```python
from build123d import *

# Parameters (mm, degrees)
BOSS_EXTRUDE1_DEPTH = 2
FILLET1_R           = 1
SKETCH2_R           = 6
CUT_EXTRUDE1_DEPTH  = 19.418740456


with BuildPart() as part:
    # Sketch1 → Boss-Extrude1 (new body)
    with BuildSketch(Plane(origin=(0, 0, 0), x_dir=(1, 0, 0), z_dir=(0, 1, 0))):
        Polygon((0, -15), (-10.5, -15), (-10.5, 15), (10.5, 15), (10.5, -15), align=None)
    extrude(amount=BOSS_EXTRUDE1_DEPTH)

    # Fillet1
    fillet1_edges = [part.edges().sort_by_distance(p)[0] for p in [
        (-10.5, 1, 15),
        (-10.5, 1, -15),
    ]]
    fillet(fillet1_edges, radius=FILLET1_R)

    # Sketch2 → Cut-Extrude1 (cut, through all)
    with BuildSketch(Plane(origin=(0, 2, 0), x_dir=(1, 0, 0), z_dir=(0, 1, 0))):
        with Locations(Location((-1.5, 0, 0), (0, 0, 270))):
            Circle(SKETCH2_R)
    extrude(amount=-CUT_EXTRUDE1_DEPTH, mode=Mode.SUBTRACT)


solid = part.part
```
The model under review builds one solid part; all positions refer to its coordinate system, in mm. Round coordinates to 2 decimals unless told otherwise and drop trailing zeros. Loops run counter-clockwise (first coordinate to the right, second up) from the corner with the lowest first, then second, coordinate; pieces in that order, holes last. Notation, with made-up numbers: M 35.5,-19 L 79.5,-19 A27 ccw 79.5,0 Z; hole C 21,45 d6. An arc over 180 degrees is marked long. Put each result on its own line as item: value.
Q1. Mouldability with a two-part tool opening along X and no side actions: class faces 1 (the flat face through (10.5, 1, 0)), 2 (the cylindrical face through (-10.199, 1.014, 14.715)), 3 (the flat face through (5, 2, 0)), 4 (the cylindrical face through (0.302, 1.014, 5.723)) as released by +X, released by -X, zero draft, split by the parting line, or undercut.
Result set:
face 1: released by +X
face 2: released by -X
face 3: zero draft
face 4: undercut
Q2. Consider section C-C, the plane z = 0. Give the boundary of the cut face in (x, y).
Result set:
outline: M -10.5,0 L -7.5,0 L -7.5,2 L -10.5,2 Z; M 4.5,0 L 10.5,0 L 10.5,2 L 4.5,2 Z
Q3. Consider section A-A, the plane x = -1.5. Give the boundary of the cut face in (y, z), then the cut area to 3 significant figures.
Result set:
outline: M 0,-15 L 2,-15 L 2,-6 L 0,-6 Z; M 0,6 L 2,6 L 2,15 L 0,15 Z
area: 36.0 mm²
Q4. To check wall thickness, follow L1, parallel to X at y = 1.05, z = 0; L2, parallel to Z at x = 0.25, y = 0.2; L3, parallel to Z at x = -5.75, y = 0.6. State the ranges of each line that lie inside material, in increasing order.
Result set:
L1: x = -10.5 to -7.5, 4.5 to 10.5
L2: z = -15 to -5.74, 5.74 to 15
L3: z = -15 to -4.24, 4.24 to 15
Q5. For pin 1 (10 mm diameter, centred on x = 3.5, z = -3, fed in from +Y), flat-tipped, find the tip position at first contact; note if it passes through.
Result set:
pin 1: stops at y = 2
Q6. Consider section B-B, the plane y = 0.4. Give the boundary of the cut face in (x, z).
Result set:
outline: M -10.5,-14 A1 ccw -9.5,-15 L 10.5,-15 L 10.5,15 L -9.5,15 A1 ccw -10.5,14 Z; hole C -1.5,0 d12
